The figure shows three views and two pictorial views of one solid part (mm, origin at its lowest corner). Answer the questions. A direction names the side the tool comes from. Coordinates: 2 decimals unless noted, no trailing zeros. Loops run counter-clockwise (first coordinate to the right, second up) from the corner with the lowest first, then second, coordinate; pieces in that order, holes last. Notation, with made-up numbers: (-31, -21) - (-6, -21) arc R8 cw to (-6, -9) - close; hole circle Ø5 at (-31.75, 30.5). An arc over 180 degrees is marked (long way). Return JSON: item names as keys, results as strings. Group by question number.
1. Section A-A (y = 4) is taken. Write down the section's boundary in (x, z) (1 decimal), and give its area (3 significant figures).
2. The mould has two halves that part along X. Classify the marked faces 3, 4 and 5: pulls with the +X half, pulls with the -X half, needs draft (parallel to the pull), parting line crosses it, or undercut.
3. Section B-B (z = 8.75) is taken. Write down the section's boundary in (x, y), and give its area (3 significant figures).
4. Section D-D (x = 7) is taken. Write down the section's boundary in (y, z).
5. Each of these flat-tipped pins is pushed along its axis until it touches: P1, Ø6, axis at y = 9.5, z = 2, coming from the -X side; P2, Ø1.7, axis at x = 25.908, z = 2.032, coming from the -Y side; P3, Ø5, axis at x = 21.5, z = 11.5, coming from the +Y side; P4, Ø6, axis at x = 24, z = 9, coming from the +Y side. Where does it stop, or does it pass through?
6. Section C-C (z = 5) is taken. Write down the section's boundary in (x, y).
7. Which of the six approach directions +Z, -Z, +X, -X, +Y, -Y give full straight-line access (tool end or side, diameter ignored) to the marked faces 1 and 2?
8. Find the intervals of material crossed by line 1 along Y through (x, z) = (17.5, 8.25); line 2 along X through (y, z) = (6, 6.75) (1 decimal); line 3 along X through (y, z) = (10.75, 7.25), in increasing order.
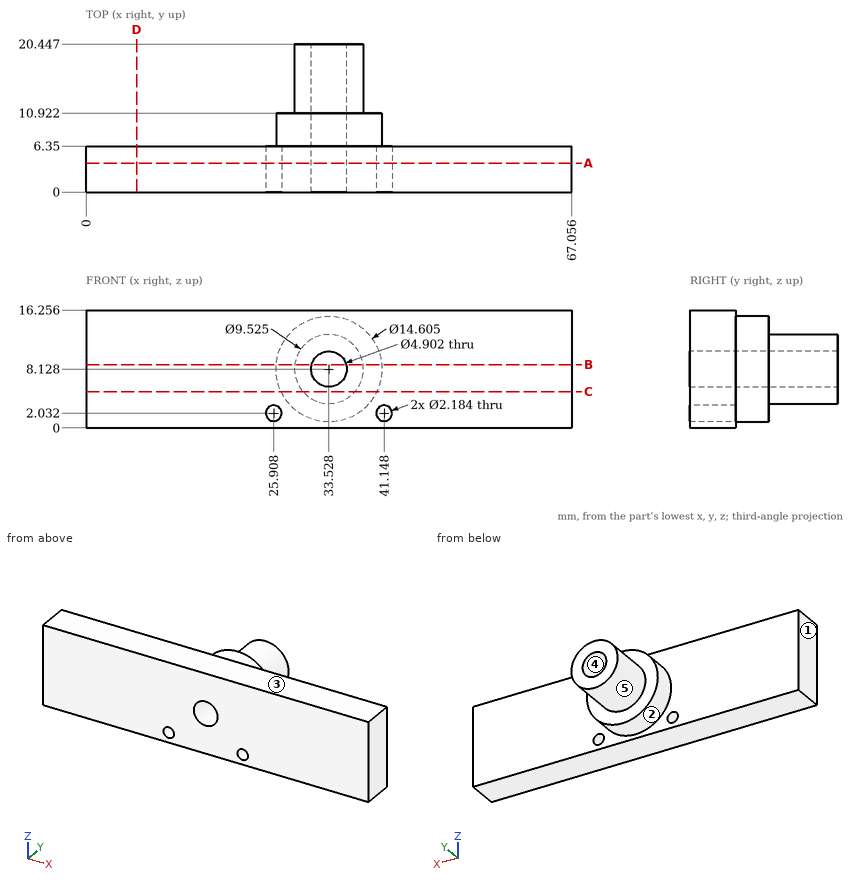
The answers:
{
 "1": {"outline": "(0, 0) - (67.1, 0) - (67.1, 16.3) - (0, 16.3) - close; hole circle Ø2.2 at (25.9, 2); hole circle Ø4.9 at (33.5, 8.1); hole circle Ø2.2 at (41.1, 2)", "area": "1,060 mm2"},
 "2": {"face 3": "needs draft", "face 4": "undercut", "face 5": "parting line crosses it"},
 "3": {"outline": "(0, 0) - (31.16, 0) - (31.16, 20.45) - (28.81, 20.45) - (28.81, 10.92) - (26.25, 10.92) - (26.25, 6.35) - (0, 6.35) - close; (35.9, 0) - (67.06, 0) - (67.06, 6.35) - (40.8, 6.35) - (40.8, 10.92) - (38.25, 10.92) - (38.25, 20.45) - (35.9, 20.45) - close", "area": "485 mm2"},
 "4": {"outline": "(0, 0) - (6.35, 0) - (6.35, 16.26) - (0, 16.26) - close"},
 "5": {"P1": "stops at x = 26.93", "P2": "passes through", "P3": "stops at y = 6.35", "P4": "stops at y = 10.92"},
 "6": {"outline": "(0, 0) - (67.06, 0) - (67.06, 6.35) - (40.13, 6.35) - (40.13, 10.92) - (37.12, 10.92) - (37.12, 20.45) - (29.94, 20.45) - (29.94, 10.92) - (26.93, 10.92) - (26.93, 6.35) - (0, 6.35) - close"},
 "7": {"face 1": "+Z, -Z, -X, +Y, -Y", "face 2": "+Y"},
 "8": {"line 1": "y = 0 to 6.35", "line 2": "x = 0 to 31.5, 35.6 to 67.1", "line 3": "x = 26.28 to 31.24, 35.82 to 40.78"}
}
